Check sheet for the modelled part. Datum: model origin and axes. Units: mm. A direction names the side the tool comes from. Round coordinates to 2 decimals unless told otherwise and drop trailing zeros. Order: outer loops, then holes, each group sorted by start corner. A loop starts at its lowest first (then second) coordinate and runs counter-clockwise, first axis right, second up.
(1) Sectioned sample at D-D, the plane y = 15. Enter the section's corners in (x, z), and give its area (3 significant figures).
(2) Depth check by flat-ended pin: pin 1 (1 mm diameter, centred on x = -5.5, y = -49.5, fed in from +Z); pin 2 (6 mm diameter, centred on x = 0, y = 43.5, fed in from -Z); pin 3 (2 mm diameter, centred on x = 0, y = 39.51, fed in from +Z); pin 4 (3 mm diameter, centred on x = -6, y = -53, fed in from -Z). Enter the tip coordinate at first touch or a pass-through.
(3) Sectioned sample at C-C, the plane z = -25.5. Enter the section's corners in (x, y), and give its area (4 significant figures).
(4) Mould release check, pull along Y, two halves, no side actions. Record for faces 1 (the flat face through (3.5, 30.05, -0.48)), 2 (the flat face through (-7.5, 37, 0)), 3 (the cylindrical face through (0.01, -42.83, -30.9)): released by +Y, released by -Y, zero draft, split by the parting line, or undercut.
(5) Tool access check on faces 4 (the flat face through (2.5, 13, 0)), 5 (the cylindrical face through (5.79, -24.28, -17.76)), 6 (the flat face through (-2.5, 13, 0)), 7 (the cylindrical face through (0.04, 59.14, -0.48)). Record the directions out of +Z, -Z, +X, -X, +Y, -Y that give a thin tool (end or side, any length) a straight path to the whole face; none if there is none.
(6) Thickness scan on probe 1 along X at (y, z) = (-12.5, -22.5); probe 2 along Y at (x, z) = (0, 1.45); probe 3 along X at (y, z) = (-35, -10.5). Record the ranges inside material, lowest first.
(7) Sectioned sample at A-A, the plane y = -46. Enter the section's corners in (x, z).
(8) Sectioned sample at B-B, the plane z = -9. Enter the section's corners in (x, y).
```python
from build123d import *

# Parameters (mm, degrees)
EXTRUDE_1_DEPTH          = 2
EXTRUDE_1_DEPTH_BACK     = 2
SKETCH_6_W               = 37
SKETCH_6_H               = 3
EXTRUDE_2_DEPTH          = 7.5
EXTRUDE_2_DEPTH_BACK     = 7.5
EXTRUDE_4_DEPTH          = 1
EXTRUDE_4_DEPTH_BACK     = 1
FILLET_1_R               = 3
EXTRUDE_8_DEPTH          = 17
EXTRUDE_8_DEPTH_BACK     = 17
CUT_EXTRUDE_3_DEPTH      = 17.5
CUT_EXTRUDE_3_DEPTH_BACK = 17.5
FILLET_7_R               = 3
FILLET_8_R               = 3
FILLET_9_R               = 3
FILLET_10_R              = 3
SKETCH_21_W              = 5
SKETCH_21_H              = 10
CUT_EXTRUDE_4_DEPTH      = 4
CUT_EXTRUDE_5_DEPTH      = 1
CUT_EXTRUDE_5_DEPTH_BACK = 2
SKETCH_23_R              = 1.25
CUT_EXTRUDE_6_DEPTH      = 13


with BuildPart() as part:
    # Sketch 1 → Extrude 1 (new body, two sides)
    with BuildSketch(Plane.XY) as extrude_1_sk:
        with BuildLine():
            Line((7.5, 8), (7.5, 55))
            ThreePointArc((7.5, 55), (0, 62.5), (-7.5, 55))
            Line((-7.5, 55), (-7.5, 8))
            Line((-7.5, 8), (7.5, 8))
        make_face()
    extrude(amount=EXTRUDE_1_DEPTH)
    extrude(extrude_1_sk.sketch, amount=-EXTRUDE_1_DEPTH_BACK)

    # Sketch 6 → Extrude 2 (add, two sides)
    with BuildSketch(Plane(origin=(0, 0, 0), x_dir=(0, 0, -1), z_dir=(1, 0, 0))) as extrude_2_sk:
        with Locations((16.5, 6.5)):
            Rectangle(SKETCH_6_W, SKETCH_6_H)
    extrude(amount=EXTRUDE_2_DEPTH)
    extrude(extrude_2_sk.sketch, amount=-EXTRUDE_2_DEPTH_BACK)

    # Sketch 8 → Extrude 4 (add, two sides)
    with BuildSketch(Plane(origin=(0, 0, 0), x_dir=(0, 0, -1), z_dir=(1, 0, 0))) as extrude_4_sk:
        with BuildLine():
            Line((1, 5), (35, 5))
            Line((35, 5), (35, -14.904717451))
            ThreePointArc((35, -14.904717451), (30.055498448, -45.958152709), (18, -75))
            ThreePointArc((18, -75), (5.944501552, -45.958152709), (1, -14.904717451))
            Line((1, -14.904717451), (1, 5))
        make_face()
    extrude(amount=EXTRUDE_4_DEPTH)
    extrude(extrude_4_sk.sketch, amount=-EXTRUDE_4_DEPTH_BACK)

    # Fillet 1
    fillet_1_edges = [part.edges().sort_by_distance(p)[0] for p in [
        (0, -75, -18),
    ]]
    fillet(fillet_1_edges, radius=FILLET_1_R)

    # Sketch 19 → Extrude 8 (add, two sides)
    with BuildSketch(Plane.XY.offset(-18)) as extrude_8_sk:
        with BuildLine():
            Line((6.5, 5), (5.5, 5))
            ThreePointArc((5.5, 5), (5.47282517, -33.328822067), (2, -71.5))
            Line((2, -71.5), (3, -71.5))
            ThreePointArc((3, -71.5), (6.537897336, -33.331799225), (6.5, 5))
        make_face()
        with BuildLine():
            Line((-3, -71.5), (-2, -71.5))
            ThreePointArc((-2, -71.5), (-5.47282517, -33.328822067), (-5.5, 5))
            Line((-5.5, 5), (-6.5, 5))
            ThreePointArc((-6.5, 5), (-6.537897336, -33.331799225), (-3, -71.5))
        make_face()
    extrude(amount=EXTRUDE_8_DEPTH)
    extrude(extrude_8_sk.sketch, amount=-EXTRUDE_8_DEPTH_BACK)

    # Sketch 20 → Cut-Extrude 3 (cut, two sides)
    with BuildSketch(Plane(origin=(0, 0, 0), x_dir=(0, 0, -1), z_dir=(1, 0, 0))) as cut_extrude_3_sk:
        with BuildLine():
            Line((1, -14.904717451), (1, -76.940462962))
            Line((1, -76.940462962), (35, -76.940462962))
            Line((35, -76.940462962), (35, -14.904717451))
            ThreePointArc((35, -14.904717451), (30.055498448, -45.958152709), (18, -75))
            ThreePointArc((18, -75), (5.944501552, -45.958152709), (1, -14.904717451))
        make_face()
    extrude(amount=CUT_EXTRUDE_3_DEPTH, mode=Mode.SUBTRACT)
    extrude(cut_extrude_3_sk.sketch, amount=-CUT_EXTRUDE_3_DEPTH_BACK, mode=Mode.SUBTRACT)

    # Fillet 7
    fillet_7_edges = [part.edges().sort_by_distance(p)[0] for p in [
        (2.5, -71.5, -16.104414556),
    ]]
    fillet(fillet_7_edges, radius=FILLET_7_R)

    # Fillet 8
    fillet_8_edges = [part.edges().sort_by_distance(p)[0] for p in [
        (2.5, -71.5, -19.895585444),
    ]]
    fillet(fillet_8_edges, radius=FILLET_8_R)

    # Fillet 9
    fillet_9_edges = [part.edges().sort_by_distance(p)[0] for p in [
        (-2.5, -71.5, -16.104414556),
    ]]
    fillet(fillet_9_edges, radius=FILLET_9_R)

    # Fillet 10
    fillet_10_edges = [part.edges().sort_by_distance(p)[0] for p in [
        (-2.5, -71.5, -19.895585444),
    ]]
    fillet(fillet_10_edges, radius=FILLET_10_R)

    # Sketch 21 → Cut-Extrude 4 (cut)
    with BuildSketch(Plane.XY.offset(2)):
        with Locations((-5, 13)):
            Rectangle(SKETCH_21_W, SKETCH_21_H)
        with Locations((5, 13)):
            Rectangle(SKETCH_21_W, SKETCH_21_H)
    extrude(amount=-CUT_EXTRUDE_4_DEPTH, mode=Mode.SUBTRACT)

    # Sketch 3 → Cut-Extrude 5 (cut, two sides)
    with BuildSketch(Plane.XY) as cut_extrude_5_sk:
        with BuildLine():
            Line((-2.106194146, 57.35480611), (-4.932538983, 40.323847539))
            ThreePointArc((-4.932538983, 40.323847539), (-5, 39.50527611), (-4.932538983, 38.686704682))
            Line((-4.932538983, 38.686704682), (-2.106194146, 21.65574611))
            ThreePointArc((-2.106194146, 21.65574611), (0, 19.87027611), (2.106194146, 21.65574611))
            Line((2.106194146, 21.65574611), (4.932538983, 38.686704682))
            ThreePointArc((4.932538983, 38.686704682), (5, 39.50527611), (4.932538983, 40.323847539))
            Line((4.932538983, 40.323847539), (2.106194146, 57.35480611))
            ThreePointArc((2.106194146, 57.35480611), (0, 59.14027611), (-2.106194146, 57.35480611))
        make_face()
    extrude(amount=CUT_EXTRUDE_5_DEPTH, mode=Mode.SUBTRACT)
    extrude(cut_extrude_5_sk.sketch, amount=-CUT_EXTRUDE_5_DEPTH_BACK, mode=Mode.SUBTRACT)

    # Sketch 23 → Cut-Extrude 6 (cut)
    with BuildSketch(Plane(origin=(0, 0, -2), x_dir=(-1, 0, 0), z_dir=(0, 0, -1))):
        with Locations((0, 39.50527611)):
            Circle(SKETCH_23_R)
    extrude(amount=-CUT_EXTRUDE_6_DEPTH, mode=Mode.SUBTRACT)


solid = part.part
```
Derived:
1. outline: (-2.5, -2) - (2.5, -2) - (2.5, 2) - (-2.5, 2) - close
1. area: 20.0 mm2
2. pin 1: stops at z = -6.84
2. pin 2: stops at z = 1
2. pin 3: passes through
2. pin 4: stops at z = -28.3
3. outline: (-7.5, 5) - (-6.5, 5) arc R410.48 ccw to (-4.52, -59.32) - (-3.48, -59.32) arc R425.92 cw to (-5.5, 5) - (-1, 5) - (-1, -59.32) - (1, -59.32) - (1, 5) - (5.5, 5) arc R425.92 cw to (3.48, -59.32) - (4.52, -59.32) arc R410.48 ccw to (6.5, 5) - (7.5, 5) - (7.5, 8) - (-7.5, 8) - close
3. area: 308.5 mm2
4. face 1: undercut
4. face 2: zero draft
4. face 3: released by -Y
5. face 4: +Z, -Z, +X
5. face 5: +Z, -Z
5. face 6: +Z, -Z, -X
5. face 7: -Z
6. probe 1: x = -6.96 to -5.92, -1 to 1, 5.92 to 6.96
6. probe 2: y = 5 to 38.26, 40.76 to 62.5
6. probe 3: x = -6.46 to -5.39, -1 to 1, 5.39 to 6.46
7. outline: (-5.76, -30.04) - (-4.7, -30.04) - (-4.7, -5.96) - (-5.76, -5.96) - close; (-1, -30.04) - (1, -30.04) - (1, -5.96) - (-1, -5.96) - close; (4.7, -30.04) - (5.76, -30.04) - (5.76, -5.96) - (4.7, -5.96) - close
8. outline: (-7.5, 5) - (-6.5, 5) arc R410.48 ccw to (-4.93, -55.41) - (-3.89, -55.41) arc R425.92 cw to (-5.5, 5) - (-1, 5) - (-1, -55.41) - (1, -55.41) - (1, 5) - (5.5, 5) arc R425.92 cw to (3.89, -55.41) - (4.93, -55.41) arc R410.48 ccw to (6.5, 5) - (7.5, 5) - (7.5, 8) - (-7.5, 8) - close
